Check sheet for the drawn part. Datum: minimum x, y, z corner. Units: mm. A direction names the side the tool comes from. Coordinates: 2 decimals unless noted, no trailing zeros. Write each loop counter-clockwise with the first axis right and the second up, starting at its lowest first coordinate (ties: lowest second). Pieces come first, ordered by that corner, then holes. Notation, with made-up numbers: (-19, -31.5) - (1, -31.5) arc R3 ccw to (1, -26.5) - close; hole circle Ø9 at (21.5, 46.5). An arc over 180 degrees is marked (long way). Write each question's results on one line, items separated by ' | '.
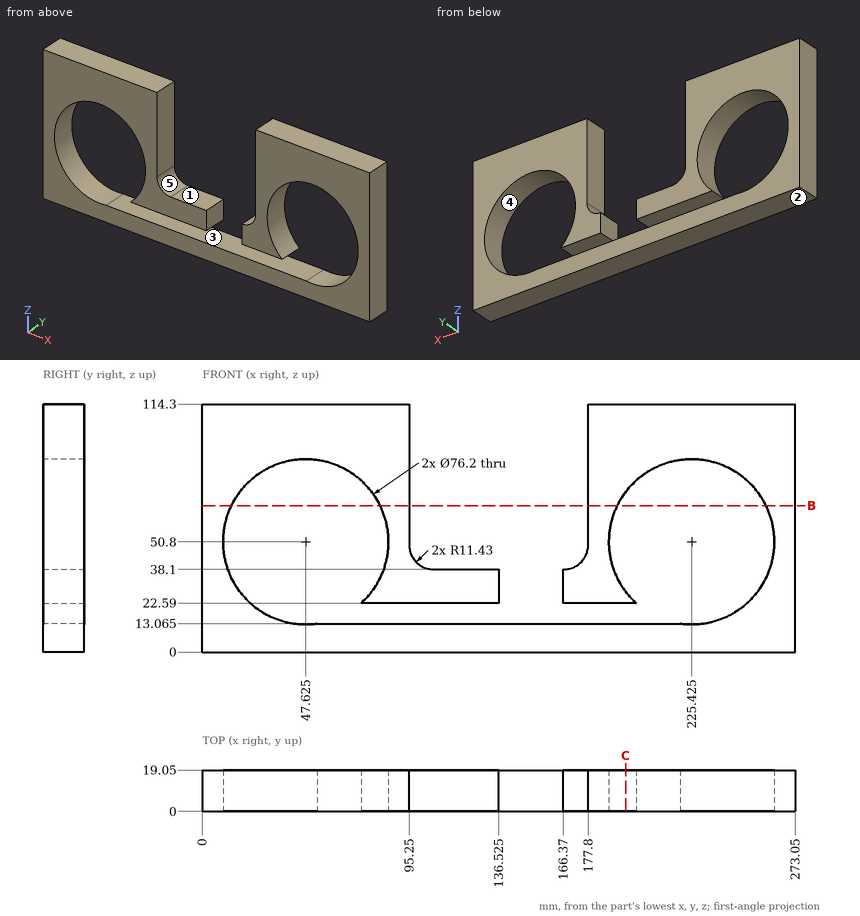
1. Material ranges on L1, parallel to X at y = 6.75, z = 50.8 (3 decimals); L2, parallel to X at y = 12.5, z = 99; L3, parallel to Z at x = 183.5, y = 6 (1 decimal), recorded low to high. Write a range as [from, to].
Values follow:
L1: x = [0, 9.525], [85.725, 95.25], [177.8, 187.325], [263.525, 273.05] | L2: x = [0, 95.25], [177.8, 273.05] | L3: z = [0, 13.1], [22.6, 114.3]
2. Go/stop test with a flat-tipped pin: pin 1 (3 mm diameter, centred on y = 16.5, z = 41, fed in from -X). Record where the tip stops, or that it passes through.
Values follow:
pin 1: stops at x = 0
3. Sectioned sample at B-B (z = 67.5). Record the cut outline in (x, y), then the cut area to 3 significant figures.
Values follow:
outline: (0, 0) - (13.38, 0) - (13.38, 19.05) - (0, 19.05) - close; (81.87, 0) - (95.25, 0) - (95.25, 19.05) - (81.87, 19.05) - close; (177.8, 0) - (191.18, 0) - (191.18, 19.05) - (177.8, 19.05) - close; (259.67, 0) - (273.05, 0) - (273.05, 19.05) - (259.67, 19.05) - close | area: 1,020 mm^2
4. Access from +Z, -Z, +X, -X, +Y, -Y to the whole of each face (thin tool, end or side, straight path). Record for the marked faces 4 and 5.
Values follow:
face 4: +Y, -Y | face 5: +Z, +Y, -Y
5. Sectioned sample at C-C (x = 195). Give the number of separate pieces and of enclosed holes in the cut face, then the cut area to 3 significant figures.
Values follow:
separate pieces: 3 | enclosed holes: 0 | area: 1,120 mm^2
6. Draft check along Z on the marked faces 1, 2 and 3. Enter one of: pulls with the +Z half, pulls with the -Z half, needs draft (parallel to the pull), parting line crosses it, or undercut.
Values follow:
face 1: pulls with the +Z half | face 2: pulls with the -Z half | face 3: undercut
